Work out the finished part from the listing and answer in its coordinate system (mm). Face numbers are marked on the shaded views. Coordinates: 2 decimals unless noted, no trailing zeros. Loops run counter-clockwise (first coordinate to the right, second up) from the corner with the lowest first, then second, coordinate; pieces in that order, holes last. Notation, with made-up numbers: (2.5, 47) - (25.5, 47) arc R26 cw to (25.5, 82) - close; hole circle Ø9 at (73.5, 12). An arc over 180 degrees is marked (long way). Write each question's results on one line, items separated by ' | '. Start each with the question number.
Item 1: Section C-C, the plane x = 50.5 is taken. Write down the section's boundary in (y, z), plus the area to 3 significant figures.
Item 2: Each of these flat-tipped pins is pushed along its axis until it touches: pin 1 Ø5 at (y, z) = (35.5, -40) entering from +X; pin 2 Ø10 at (x, z) = (42.5, -13.5) entering from -Y; pin 3 Ø4.5 at (y, z) = (12.5, -41.5) entering from -X; pin 4 Ø5 at (y, z) = (43.5, -109) entering from -X. Where does it stop, or does it pass through?
Item 3: Consider probe 1 along Z at (x, y) = (111, 0.9); probe 2 along Z at (x, y) = (63, 53); probe 3 along Z at (x, y) = (80, 103.5). Determine where each line is inside the solid, lowest interval first. Write a range as [from, to].
Item 4: Section B-B, the plane y = 59.6 is taken. Write down the section's boundary in (x, z), plus the area to 3 significant figures.
Item 5: For a pull along Y with two mould halves and no side action, classify the marked faces 1, 2, 3 and 4 as +Y half, -Y half, draft (parallel to the pull), parting line (faces both ways), or undercut.
Item 6: Section A-A, the plane z = -64 is taken. Write down the section's boundary in (x, y), plus the area to 3 significant figures.
Item 7: Section D-D, the plane z = -45 is taken. Write down the section's boundary in (x, y), plus the area to 3 significant figures.
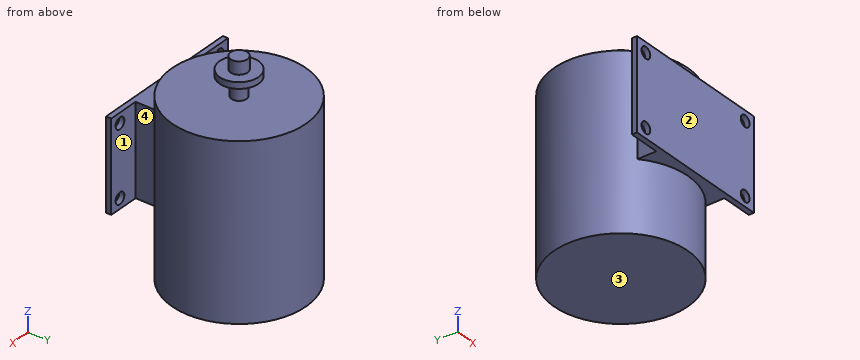
Autodesk Inventor part; units mm, degrees
ref_plane "YZ Plane" through (0, 0, 0) normal (1, 0, 0) x (0, 1, 0)
ref_plane "XZ Plane" through (0, 0, 0) normal (0, 1, 0) x (-1, 0, 0)
ref_plane "XY Plane" through (0, 0, 0) normal (0, 0, 1) x (1, 0, 0)
sketch "Sketch1" plane through (0, 0, 0) normal (0, 1, 0) x (-1, 0, 0)
  line L0 (0, 0) -> (-120, 0)
  line L1 (-120, 0) -> (-120, -72)
  line L2 (-120, -72) -> (0, -72)
  line L3 (0, -72) -> (0, 0)
  circle A0 centre (-9, -8) radius 4.5
  circle A1 centre (-111, -8) radius 4.5
  circle A2 centre (-9, -64) radius 4.5
  circle A3 centre (-111, -64) radius 4.5
  dimension "d0" = 120
  dimension "d1" = 72
  dimension "d2" = 9
  dimension "d3" = 9
  dimension "d4" = 9
  dimension "d5" = 9
extrude "Extrusion1" add sketch "Sketch1" along normal blind 4.1
sketch "Sketch2" plane through (0, 4.1, 0) normal (0, 1, 0) x (1, 0, 0)
  line L0 (0, 0) -> (120, 0)
  line L1 (120, 72) -> (0, 72)
  line L2 (25, 0) -> (95, 0)
  line L3 (95, 0) -> (95, 72)
  line L4 (95, 72) -> (25, 72)
  line L5 (25, 72) -> (25, 0)
  dimension "d8" = 70
extrude "Extrusion2" add sketch "Sketch2" along normal blind 53.5
sketch "Sketch3" plane through (0, 0, 0) normal (0, 0, 1) x (1, 0, 0)
  circle A0 centre (60, 59.6) radius 53.5
  point P0 (0, 0)
  dimension "d11" = 107
extrude "Extrusion3" add sketch "Sketch3" along normal blind 8.5 and the other way blind 128
sketch "Sketch4" plane through (60, 59.6, 8.5) normal (0, 0, 1) x (1, 0, 0)
  circle A0 centre (0, 0) radius 6
  point P0 (-60, -59.6)
  dimension "d16" = 12
extrude "Extrusion4" add sketch "Sketch4" along normal blind 15
sketch "Sketch5" plane through (60, 59.6, 23.5) normal (0, 0, 1) x (1, 0, 0)
  circle A0 centre (0, 0) radius 15.5
  point P0 (-60, -59.6)
  dimension "d19" = 31
extrude "Extrusion5" add sketch "Sketch5" along normal blind 5
sketch "Sketch6" plane through (60, 59.6, 28.5) normal (0, 0, 1) x (1, 0, 0)
  circle A0 centre (0, 0) radius 6.75
  point P0 (-60, -59.6)
  dimension "d22" = 13.5
extrude "Extrusion6" add sketch "Sketch6" along normal blind 10
properties part number "BLDC BM1109 MOTOR"
Answer key:
1) outline: (0, -72) - (6.95, -72) - (6.95, -128) - (112.25, -128) - (112.25, 8.5) - (6.95, 8.5) - (6.95, 0) - (0, 0) - close; (47.35, 23.5) - (71.85, 23.5) - (71.85, 28.5) - (47.35, 28.5) - close | area: 15,000 mm^2
2) pin 1: stops at x = 108.95 | pin 2: stops at y = 0 | pin 3: stops at x = 25 | pin 4: stops at x = 8.26
3) probe 1: z = [-72, -68.5], [-59.5, -12.5], [-3.5, 0] | probe 2: z = [-128, 8.5], [23.5, 28.5] | probe 3: z = [-128, 8.5]
4) outline: (6.5, -128) - (113.5, -128) - (113.5, 8.5) - (66, 8.5) - (66, 23.5) - (75.5, 23.5) - (75.5, 28.5) - (66.75, 28.5) - (66.75, 38.5) - (53.25, 38.5) - (53.25, 28.5) - (44.5, 28.5) - (44.5, 23.5) - (54, 23.5) - (54, 8.5) - (6.5, 8.5) - close | area: 15,100 mm^2
5) face 1: undercut | face 2: -Y half | face 3: draft | face 4: undercut
6) outline: (0, 0) - (4.5, 0) - (4.5, 4.1) - (0, 4.1) - close; (13.5, 0) - (106.5, 0) - (106.5, 4.1) - (95, 4.1) - (95, 19.14) arc R53.5 ccw (long way) to (25, 19.14) - (25, 4.1) - (13.5, 4.1) - close; (115.5, 0) - (120, 0) - (120, 4.1) - (115.5, 4.1) - close | area: 9,840 mm^2
7) outline: (0, 0) - (120, 0) - (120, 4.1) - (95, 4.1) - (95, 19.14) arc R53.5 ccw (long way) to (25, 19.14) - (25, 4.1) - (0, 4.1) - close | area: 9,910 mm^2
